```python
from build123d import *

# Parameters (mm, degrees)
BOSS_EXTRUDE1_DEPTH   = 7
FILLET1_R             = 1
FILLET2_R             = 1
FILLET3_R             = 1
CUT_EXTRUDE1_DEPTH    = 6
F_4_0MM_DOWEL_HOLE1_D = 4.5


with BuildPart() as part:
    # Sketch1 → Boss-Extrude1 (new body)
    with BuildSketch(Plane.XY):
        with BuildLine():
            Line((51, 0), (51, 25.5))
            ThreePointArc((51, 25.5), (49.182412553, 33.297587625), (44.104318796, 39.487818693))
            ThreePointArc((44.104318796, 39.487818693), (44.100505812, 39.494158329), (44.096690854, 39.500496777))
            Line((44.096690854, 39.500496777), (47.63222476, 43.036030683))
            ThreePointArc((47.63222476, 43.036030683), (48.118470522, 47.63222476), (43.522276444, 48.118470522))
            Line((43.522276444, 48.118470522), (39.986742538, 44.582936616))
            ThreePointArc((39.986742538, 44.582936616), (6.956213947, 44.043786053), (6.417063384, 11.013257462))
            Line((6.417063384, 11.013257462), (2.881529478, 7.477723556))
            ThreePointArc((2.881529478, 7.477723556), (3.36777524, 2.881529478), (7.963969317, 3.36777524))
            Line((7.963969317, 3.36777524), (11.499503223, 6.903309146))
            ThreePointArc((11.499503223, 6.903309146), (21.530362571, 3.603949385), (32, 4.978942549))
            Line((32, 4.978942549), (32, 0))
            Line((32, 0), (51, 0))
        make_face()
    extrude(amount=BOSS_EXTRUDE1_DEPTH)

    # Fillet1
    # the kernel refuses this fillet: 1 mm, written as the material it adds along each edge
    with BuildSketch(Plane(origin=(44.096690854, 39.500496777, 0), x_dir=(0.7715576110634285, -0.6361594554905989, 0), z_dir=(0, 0, 1))) as fillet1_piece_1:
        with BuildLine():
            CenterArc((1.100766551, 0.999676081), FILLET1_R, 174.506032256, 94.03559873)
            Line((0.105360267, 1.095417035), (0.005819639, 1.104991131))
            Line((0.005819639, 1.104991131), (-0.099540628, 0.009574095))
            Line((-0.099540628, 0.009574095), (-0.033285789, -0.0942977))
            ThreePointArc((-0.033285789, -0.0942977), (0.017424165, -0.104868941), (1.072770899, -0.099967608))
            Line((1.072770899, -0.099967608), (1.075315958, 0))
        make_face()
    extrude(amount=7)
    with BuildSketch(Plane(origin=(44.104318796, 39.487818693, 0), x_dir=(0.7745037653558564, -0.6325692985354254, 0), z_dir=(0, 0, 1))) as fillet1_piece_2:
        with BuildLine():
            CenterArc((1.091469777, 0.999547102), FILLET1_R, 174.23993613, 94.03559873)
            Line((0.096518871, 1.099909926), (-0.002976219, 1.109946208))
            ThreePointArc((-0.002976219, 1.109946208), (-0.113422726, 0.015030304), (-0.033782013, -0.094121069))
            Line((-0.033782013, -0.094121069), (0.003009305, -0.09995471))
            ThreePointArc((0.003009305, -0.09995471), (0.530688363, -0.092013175), (1.058367421, -0.09995471))
            Line((1.058367421, -0.09995471), (1.061376726, 0))
        make_face()
    extrude(amount=7)

    # Fillet2
    fillet2_edges = [part.edges().sort_by_distance(p)[0] for p in [
        (11.499503223, 6.903309146, 3.5),
        (6.417063384, 11.013257462, 3.5),
        (39.986742538, 44.582936616, 3.5),
    ]]
    fillet(fillet2_edges, radius=FILLET2_R)

    # Fillet3
    fillet3_edges = [part.edges().sort_by_distance(p)[0] for p in [
        (32, 4.978942549, 3.5),
    ]]
    fillet(fillet3_edges, radius=FILLET3_R)

    # Sketch2 → Cut-Extrude1 (cut)
    with BuildSketch(Plane.XY.offset(7)):
        with BuildLine():
            Line((33, 0), (33, 3.389836053))
            ThreePointArc((33, 3.389836053), (32.194148238, 5.146743671), (30.28668256, 5.459307466))
            ThreePointArc((30.28668256, 5.459307466), (2.151192178, 34.39520823), (41.992282379, 40.84344083))
            ThreePointArc((41.992282379, 40.84344083), (48.304075384, 32.522702207), (50, 22.217496636))
            Line((50, 22.217496636), (50, 0))
            Line((50, 0), (33, 0))
        make_face()
    extrude(amount=-CUT_EXTRUDE1_DEPTH, mode=Mode.SUBTRACT)

    # Ø4.0mm Dowel Hole1 (through all)
    with Locations(Plane(origin=(0, 0, 0), x_dir=(-1, 0, 0), z_dir=(0, 0, -1))):
        with Locations((-5.422749398, 5.422749398), (-45.577250602, 45.577250602)):
            Hole(F_4_0MM_DOWEL_HOLE1_D / 2)


solid = part.part
```
Work out the finished part from the listing and answer in its coordinate system (mm). A direction names the side the tool comes from. Coordinates: 2 decimals unless noted, no trailing zeros. Write each loop counter-clockwise with the first axis right and the second up, starting at its lowest first coordinate (ties: lowest second). Pieces come first, ordered by that corner, then holes. Notation, with made-up numbers: (-37, 73.25) - (9, 73.25) arc R29 cw to (9, 112.25) - close; hole circle Ø4 at (-26, -37). An arc over 180 degrees is marked (long way). Answer as a JSON object with one key per item and string values.
Q1. Find section D-D (x = 36). Write down the section's boundary in (y, z).
Results list:
{"outline": "(0, 0) - (47.6, 0) - (47.6, 7) - (46.42, 7) - (46.42, 1) - (0, 1) - close"}
Q2. Find section A-A (x = 23.75). Write down the section's boundary in (y, z), plus the area to 3 significant figures.
Results list:
{"outline": "(3.5, 0) - (51, 0) - (51, 7) - (50, 7) - (50, 1) - (4.5, 1) - (4.5, 7) - (3.5, 7) - close", "area": "59.5 mm^2"}
Q3. Find section C-C (y = 32). Write down the section's boundary in (x, z).
Results list:
{"outline": "(0.48, 0) - (49.76, 0) - (49.76, 7) - (48.52, 7) - (48.52, 1) - (1.5, 1) - (1.5, 7) - (0.48, 7) - close"}
Q4. Find section B-B (z = 3.25). Write down the section's boundary in (x, y), plus the area to 3 significant figures.
Results list:
{"outline": "(2.88, 7.48) arc R3.27 ccw to (7.96, 3.37) - (10.96, 6.36) arc R1 cw to (12.15, 6.52) arc R23.75 ccw to (30.71, 4.54) arc R1 cw to (32, 3.59) - (32, 0) - (33, 0) - (33, 3.39) arc R2.06 ccw to (30.29, 5.46) arc R22.75 cw (long way) to (41.99, 40.84) arc R21.71 cw to (50, 22.22) - (50, 0) - (51, 0) - (51, 25.5) arc R17.63 ccw to (44.93, 38.82) arc R1 cw to (44.87, 40.28) - (47.63, 43.04) arc R3.27 ccw to (43.52, 48.12) - (40.66, 45.25) arc R1 cw to (39.3, 45.21) arc R23.75 ccw to (5.79, 11.7) arc R1 cw to (5.75, 10.34) - close; hole circle Ø4.5 at (5.42, 5.42); hole circle Ø4.5 at (45.58, 45.58)", "area": "216 mm^2"}
Q5. Given pin 1 Ø24.5 at (x, y) = (15, 29) entering from +Z; pin 2 Ø3 at (y, z) = (8.5, 3) entering from -X; pin 3 Ø1.5 at (x, z) = (12.5, 3.5) entering from +Y, each flat-ended and moving along its own axis, determine where each tip first touches the part or whether it passes through.
Results list:
{"pin 1": "stops at z = 1", "pin 2": "stops at x = 2.56", "pin 3": "stops at y = 48.55"}
Q6. Consider L1, parallel to X at y = 48, z = 4; L2, parallel to Y at x = 7, z = 6.25; L3, parallel to Y at x = 3.5, z = 0.5. Determine where each line is inside the solid, lowest interval first. Write a range as from..to.
Results list:
{"L1": "x = 12.2..14.42, 33.08..35.3, 43.4..47.77", "L2": "y = 2.56..3.82, 7.03..11.86, 42.64..44.09", "L3": "y = 2.78..4.25, 6.59..8.1, 14.84..39.66"}
Q7. For a pull along Y with two mould halves and no side action, classify faces 5 (the flat face through (41, 43, 7)), 6 (the cylindrical face through (43.8, 44.2, 3.5)), 7 (the cylindrical face through (39.997, 44.962, 3.549)), 8 (the cylindrical face through (31.58, 4.4, 3.55)) as pulls with the +Y half, pulls with the -Y half, needs draft (parallel to the pull), parting line crosses it, or undercut.
Results list:
{"face 5": "needs draft", "face 6": "undercut", "face 7": "pulls with the +Y half", "face 8": "pulls with the -Y half"}
Q8. Which of the six approach directions +Z, -Z, +X, -X, +Y, -Y give full straight-line access (tool end or side, diameter ignored) to faces 1 (the cylindrical face through (32.216, 5.13, 4.042)), 2 (the flat face through (46.234, 41.638, 3.451)), 3 (the flat face through (33, 2, 4)), 4 (the flat face through (32, 2, 3))?
Results list:
{"face 1": "+Z", "face 2": "+Z, -Z, +X", "face 3": "+Z, -Y", "face 4": "+Z, -Z, -Y"}
